from build123d import *

# Parameters (mm, degrees)
F0_R     = 10
F1_DEPTH = 30
F2_W     = 14.354546
F2_H     = 0.267448
F3_DEPTH = 12.7


with BuildPart() as f1:
    # F0 (on Top) → F1 (new body)
    with BuildSketch(Plane.XY):
        Circle(F0_R)
    extrude(amount=F1_DEPTH)

    # F2 (on Front) → F3 (cut, symmetric)
    with BuildSketch(Plane.XZ):
        with Locations((0, 10)):
            Rectangle(F2_W, F2_H)
        with Locations((0.068115, 19.866276)):
            Rectangle(F2_W, F2_H)
    extrude(amount=F3_DEPTH, both=True, mode=Mode.SUBTRACT)


solid = f1.part
The model under review builds one solid part; all positions refer to its coordinate system, in mm. A direction names the side the tool comes from. Round coordinates to 2 decimals unless told otherwise and drop trailing zeros. Write each loop counter-clockwise with the first axis right and the second up, starting at its lowest first coordinate (ties: lowest second). Pieces come first, ordered by that corner, then holes. Notation, with made-up numbers: M -27,22 L 10,22 A17 cw 10,39 Z; hole C 1.5,30 d3. An arc over 180 degrees is marked long. Answer as CSV lines item,"result". Start each with the question number.
Q1. Consider section A-A, the plane x = 0. Give the boundary of the cut face in (y, z), then the cut area to 3 significant figures.
Q2. Consider section C-C, the plane y = 1.5. Give the boundary of the cut face in (x, z).
Q3. Tool access review of faces 5 (the face through (0, 0, 9.866)), 6 (the face through (0, 0, 30)): name each direction out of +Z, -Z, +X, -X, +Y, -Y from which nothing blocks a thin tool from reaching the whole face with its end or side.
Q4. Consider section D-D, the plane x = 8. Give the boundary of the cut face in (y, z), then the cut area to 3 significant figures.
Q5. Clearance check with flat-ended pins moving along their axes: P1, Ø5, axis at y = -7, z = 8.5, coming from the +X side; P2, Ø1, axis at y = -4.5, z = 25.5, coming from the -X side; P3, Ø10, axis at x = 5.5, z = 23.5, coming from the -Y side. State where each tip first meets the part, or that it passes through.
Q6. Wall thickness on line 1 along Z through (x, y) = (-1.25, 9.25); line 2 along X through (y, z) = (7.25, 4.75): over which ranges is each line inside the solid? List them lowest first.
Q7. The part is to be moulded in two halves that separate along X. For faces 1 (the face through (0, 0, 0)), 2 (the face through (0, 0, 20)), 3 (the face through (0, 0, 19.733)), 4 (the face through (-2.17, -9.76, 14.79)), say which applies: +X half, -X half, draft (parallel to the pull), parting line (faces both ways), or undercut.
Q8. Consider section B-B, the plane y = 7.75. Give the boundary of the cut face in (x, z).
Result set:
1,outline,"M -10,0 L 10,0 L 10,9.87 L -10,9.87 Z; M -10,10.13 L 10,10.13 L 10,19.73 L -10,19.73 Z; M -10,20 L 10,20 L 10,30 L -10,30 Z"
1,area,"589 mm²"
2,outline,"M -9.89,0 L 9.89,0 L 9.89,30 L -9.89,30 Z; hole M -7.18,9.87 L 7.18,9.87 L 7.18,10.13 L -7.18,10.13 Z; hole M -7.11,19.73 L 7.25,19.73 L 7.25,20 L -7.11,20 Z"
3,face 5,"+Y, -Y"
3,face 6,"+Z, +X, -X, +Y, -Y"
4,outline,"M -6,0 L 6,0 L 6,30 L -6,30 Z"
4,area,"360 mm²"
5,P1,"stops at x = 8.93"
5,P2,"stops at x = -9.17"
5,P3,"stops at y = -9.99"
6,line 1,"z = 0 to 9.87, 10.13 to 19.73, 20 to 30"
6,line 2,"x = -6.89 to 6.89"
7,face 1,"draft"
7,face 2,"undercut"
7,face 3,"undercut"
7,face 4,"parting line"
8,outline,"M -6.32,0 L 6.32,0 L 6.32,9.87 L -6.32,9.87 Z; M -6.32,10.13 L 6.32,10.13 L 6.32,19.73 L -6.32,19.73 Z; M -6.32,20 L 6.32,20 L 6.32,30 L -6.32,30 Z"
